from build123d import *

# Parameters (mm, degrees)
SKETCH2_R           = 3.96875
BOSS_EXTRUDE1_DEPTH = 25.4
FILLET3_R           = 2.54
SKETCH3_R           = 11.303
CUT_EXTRUDE1_DEPTH  = 12.7


with BuildPart() as part:
    # Sketch2 → Boss-Extrude1 (new body)
    with BuildSketch(Plane.XY):
        with BuildLine():
            Line((16.984572795, 2.473699256), (63.5, 29.329393675))
            Line((63.5, 29.329393675), (59.055, 37.028359514))
            Line((59.055, 37.028359514), (11.202045256, 9.400443212))
            Line((11.202045256, 9.400443212), (-11.202045256, 9.400443212))
            Line((-11.202045256, 9.400443212), (-59.055, 37.028359514))
            Line((-59.055, 37.028359514), (-63.5, 29.329393675))
            Line((-63.5, 29.329393675), (-16.984572795, 2.473699256))
            ThreePointArc((-16.984572795, 2.473699256), (0, -30.51697278), (16.984572795, 2.473699256))
        make_face()
        with Locations((0, -9.649556788)):
            Circle(SKETCH2_R, mode=Mode.SUBTRACT)
    extrude(amount=BOSS_EXTRUDE1_DEPTH)

    # Fillet3
    fillet3_edges = [part.edges().sort_by_distance(p)[0] for p in [
        (61.2775, 33.178876595, 0),
        (40.242286397, 15.901546466, 0),
        (0, -30.51697278, 0),
        (-40.242286397, 15.901546466, 0),
        (40.242286397, 15.901546466, 25.4),
        (-63.5, 29.329393675, 12.7),
        (-59.055, 37.028359514, 12.7),
        (59.055, 37.028359514, 12.7),
        (63.5, 29.329393675, 12.7),
        (61.2775, 33.178876595, 25.4),
        (35.128522628, 23.214401363, 25.4),
        (0, 9.400443212, 25.4),
        (-35.128522628, 23.214401363, 25.4),
        (-61.2775, 33.178876595, 25.4),
        (-40.242286397, 15.901546466, 25.4),
        (-61.2775, 33.178876595, 0),
        (0, -30.51697278, 25.4),
        (-35.128522628, 23.214401363, 0),
        (0, 9.400443212, 0),
        (35.128522628, 23.214401363, 0),
    ]]
    fillet(fillet3_edges, radius=FILLET3_R)

    # Sketch3 → Cut-Extrude1 (cut)
    with BuildSketch(Plane.XY.offset(25.4)):
        with Locations((0, -9.649556788)):
            Circle(SKETCH3_R)
    extrude(amount=-CUT_EXTRUDE1_DEPTH, mode=Mode.SUBTRACT)


solid = part.part
Read the model definition and answer for the solid it produces. Units are mm, in the model's axes. A direction names the side the tool comes from. Give positions to 0.01 mm unless a question says otherwise; leave off trailing zeros. Write each loop counter-clockwise with the first axis right and the second up, starting at its lowest first coordinate (ties: lowest second). Pieces come first, ordered by that corner, then holes. Notation, with made-up numbers: (3.5, -19.75) - (29.5, -19.75) arc R23 cw to (29.5, 0.25) - close; hole circle Ø1 at (4.5, 4). An arc over 180 degrees is marked (long way). Answer in a Markdown table with one row per item. Add a question column.
Item 1: Section B-B, the plane z = 15.75 is taken. Write down the section's boundary in (x, y) (3 decimals), and give its area (3 significant figures).
Item 2: Flat-ended cylindrical pins translate along their axes: P1, Ø1, axis at y = 12, z = 8, coming from the +X side; P2, Ø8, axis at x = -32.5, z = 21.5, coming from the -Y side; P3, Ø3, axis at y = 3.5, z = 8.5, coming from the +X side; P4, Ø6.5, axis at x = 0, y = -9.65, coming from the -Z side. Find the tip coordinate at first contact, or state that the pin passes through.
Item 3: Find the intervals of material crossed by L1, parallel to Y at x = 0, z = 7; L2, parallel to X at y = 22, z = 23.5; L3, parallel to Y at x = 7.5, z = 15.5, in increasing order.
Item 4: Determine the mould class of faces 1 (the face through (-34.4, 22, 0.8)), 2 (the face through (37.8, 15.33, 24.64)), 3 (the face through (-61.264, 33.202, 12.558)) for opening direction X: pulls with the +X half, pulls with the -X half, needs draft (parallel to the pull), parting line crosses it, or undercut.
Item 5: A tool of negligible diameter and unlimited length cuts with its end or side. For faces 4 (the face through (-62.476, 29.575, 12.842)), 5 (the face through (6.08, -0.12, 19.14)), 6 (the face through (34.348, 22.764, 12.558)), from which of +Z, -Z, +X, -X, +Y, -Y can it reach the whole face along a straight path? Write none if from no direction.
Item 6: Section A-A, the plane x = 0 is taken. Write down the section's boundary in (y, z), and give its area (3 significant figures).
Recorded:
| question | item | result |
|---|---|---|
| 1 | outline | (-62.23, 31.529) arc R2.54 ccw to (-61.3, 28.059) - (-16.985, 2.474) arc R20.867 ccw (long way) to (16.985, 2.474) - (61.3, 28.059) arc R2.54 ccw to (62.23, 31.529) - (60.325, 34.829) arc R2.54 ccw to (56.855, 35.758) - (11.202, 9.4) - (-11.202, 9.4) - (-56.855, 35.758) arc R2.54 ccw to (-60.325, 34.829) - close; hole circle Ø22.606 at (0, -9.65) |
| 1 | area | 1,920 mm2 |
| 2 | P1 | stops at x = 34.35 |
| 2 | P2 | stops at y = 9.12 |
| 2 | P3 | stops at x = 21.36 |
| 2 | P4 | passes through |
| 3 | L1 | y = -30.52 to -13.62, -5.68 to 9.4 |
| 3 | L2 | x = -50.64 to -33.19, 33.19 to 50.64 |
| 3 | L3 | y = -29.12 to -18.11, -1.19 to 9.4 |
| 4 | face 1 | undercut |
| 4 | face 2 | pulls with the +X half |
| 4 | face 3 | pulls with the -X half |
| 5 | face 4 | +Z, -Z, -X |
| 5 | face 5 | +Z |
| 5 | face 6 | +Z, -Z, +Y |
| 6 | outline | (-30.52, 2.54) arc R2.54 ccw to (-27.98, 0) - (-13.62, 0) - (-13.62, 12.7) - (-20.95, 12.7) - (-20.95, 25.4) - (-27.98, 25.4) arc R2.54 ccw to (-30.52, 22.86) - close; (-5.68, 0) - (6.86, 0) arc R2.54 ccw to (9.4, 2.54) - (9.4, 22.86) arc R2.54 ccw to (6.86, 25.4) - (1.65, 25.4) - (1.65, 12.7) - (-5.68, 12.7) - close |
| 6 | area | 620 mm2 |
